Autodesk Inventor part; units mm, degrees
ref_plane "YZ Plane" through (0, 0, 0) normal (1, 0, 0) x (0, 1, 0)
ref_plane "XZ Plane" through (0, 0, 0) normal (0, 1, 0) x (-1, 0, 0)
ref_plane "XY Plane" through (0, 0, 0) normal (0, 0, 1) x (1, 0, 0)
sketch "Skizze1" plane through (0, 0, 0) normal (0, 0, 1) x (1, 0, 0)
  circle A0 centre (0, 0) radius 11
  dimension "d0" = 22
extrude "Extrusion1" add sketch "Skizze1" along normal blind 4
sketch "Skizze2" plane through (0, 0, 4) normal (0, 0, 1) x (1, 0, 0)
  circle A0 centre (0, 0) radius 11
  circle A1 centre (0, 0) radius 4
  dimension "d3" = 8
extrude "Extrusion2" add sketch "Skizze2" along normal blind 6 contours A1
sketch "Skizze3" plane through (0, 0, 10) normal (0, 0, 1) x (1, 0, 0)
  circle A0 centre (0, 0) radius 4
  circle A1 centre (0, 0) radius 2.5
  dimension "d6" = 5
extrude "Extrusion3" add sketch "Skizze3" along normal blind 20 contours A1
sketch "Skizze4" plane through (0, 0, 0) normal (0, 0, -1) x (-1, 0, 0)
  circle A0 centre (0, 0) radius 11
  line L0 (17.5, 0) -> (-17.5, 0)
  line L1 (0, -17.5) -> (0, 17.5)
  circle A1 centre (0, 0) radius 7.5
  line L2 (6.4952, -3.75) -> (0, 0)
  line L3 (0, 0) -> (-6.4952, -3.75)
  point P0 (0, 7.5)
  dimension "d9" = 15
  dimension "d10" = 120
  dimension "d11" = 120
hole "Bohrung1" at (0, 7.5, 0) at (-6.4952, -3.75, 0) at (6.4952, -3.75, 0) direction (0, 0, 1) diameter 2.459 end through all
chamfer "Fase1" distance 0.5 angle 45 1 edges at (-2.5, 0, 30)
sketch "Skizze5" plane through (0, 0, 0) normal (1, 0, 0) x (0, 1, 0)
  line L0 (-2.5, 10) -> (2.5, 10)
  line L1 (2.5, 29.5) -> (-2.5, 29.5)
  line L2 (2.5, 10) -> (2.5, 29.5)
  line L3 (0, -4.3) -> (0, 25.8)
  line L4 (2.5, 28.7) -> (2.4, 28.7)
  line L5 (2.4, 28.7) -> (2.4, 28)
  line L6 (2.4, 28) -> (2.5, 28)
  line L7 (2.5, 28) -> (2.5, 28.7)
  point P0 (0, 0)
  dimension "d31" = 18
  dimension "d32" = 0.7
  dimension "d33" = 4.8
revolve "Umdrehung1" cut sketch "Skizze5" angle 360 about axis through (0, 0, -10) along (0, 0, 1)
chamfer "Fase3" distance 1 angle 45 1 edges at (-11, 0, 4)
properties part number "13_0204_017"
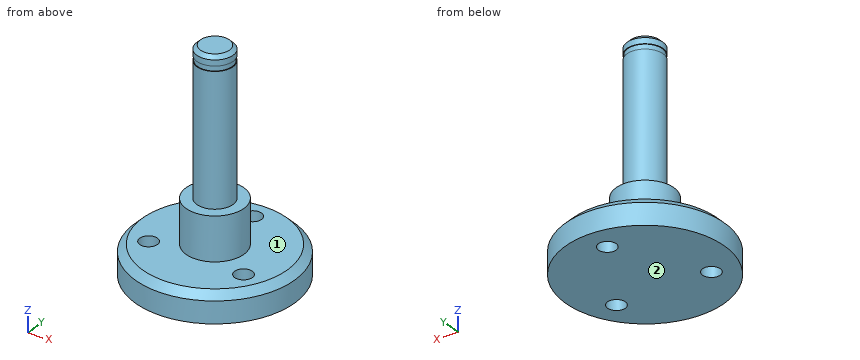
The listing builds one solid part. Answer for the finished solid, in the listing's coordinates (mm). Face numbers are marked on the shaded views. A direction names the side the tool comes from. Round coordinates to 2 decimals unless told otherwise and drop trailing zeros. Order: outer loops, then holes, each group sorted by start corner. A loop starts at its lowest first (then second) coordinate and runs counter-clockwise, first axis right, second up. Notation, with made-up numbers: (57.5, 27.5) - (116.5, 27.5) arc R28 ccw to (116.5, 66.5) - close; hole circle Ø4 at (-8.75, -22.5). An arc over 180 degrees is marked (long way). Put each result on its own line as item: value. Start each with the question number.
(1) Given P1, Ø8, axis at y = 1.5, z = 16.5, coming from the +X side; P2, Ø3, axis at x = 2.5, y = -8.5, coming from the +Z side; P3, Ø5, axis at x = 2, z = 23.5, coming from the +Y side; P4, Ø2, axis at x = -6.5, y = -3.75, coming from the -Z side, each flat-ended and moving along its own axis, determine where each tip first touches the part or whether it passes through.
(2) Find section B-B (y = 0). Give the vertices of the cut face in (x, z).
(3) Straight lines are drawn through the part: probe 1 along Y at (x, z) = (0, 1.1); probe 2 along X at (y, z) = (-3.75, 2.25); probe 3 along Z at (x, y) = (-5.25, 1.5). For each, find the intervals that lie inside material, in ascending order. Write a range as from..to.
(4) Find section D-D (z = 18.5). Give the vertices of the cut face in (x, y), plus the area to 3 significant figures.
(5) Find section C-C (z = 4.75). Give the vertices of the cut face in (x, y), plus the area to 3 significant figures.
(6) Find section A-A (x = 0). Give the vertices of the cut face in (y, z), plus the area to 3 significant figures.
(7) For the marked faces 1 and 2, determine the directions among +Z, -Z, +X, -X, +Y, -Y from which every point of the face is accessible in a straight line to the end or side of a thin tool.
Reply:
1. P1: x = 2.5
1. P2: z = 4
1. P3: y = 2.5
1. P4: through
2. outline: (-11, 0) - (11, 0) - (11, 3) - (10, 4) - (4, 4) - (4, 10) - (2.5, 10) - (2.5, 28) - (2.4, 28) - (2.4, 28.7) - (2.5, 28.7) - (2.5, 29.5) - (2, 30) - (-2, 30) - (-2.5, 29.5) - (-2.5, 28.7) - (-2.4, 28.7) - (-2.4, 28) - (-2.5, 28) - (-2.5, 10) - (-4, 10) - (-4, 4) - (-10, 4) - (-11, 3) - close
3. probe 1: -11..6.27, 8.73..11
3. probe 2: -10.34..-7.72, -5.27..5.27, 7.72..10.34
3. probe 3: 0..4
4. outline: circle Ø5 at (0, 0)
4. area: 19.6 mm^2
5. outline: circle Ø8 at (0, 0)
5. area: 50.3 mm^2
6. outline: (-11, 0) - (6.27, 0) - (6.27, 4) - (4, 4) - (4, 10) - (2.5, 10) - (2.5, 28) - (2.4, 28) - (2.4, 28.7) - (2.5, 28.7) - (2.5, 29.5) - (2, 30) - (-2, 30) - (-2.5, 29.5) - (-2.5, 28.7) - (-2.4, 28.7) - (-2.4, 28) - (-2.5, 28) - (-2.5, 10) - (-4, 10) - (-4, 4) - (-10, 4) - (-11, 3) - close; (8.73, 0) - (11, 0) - (11, 3) - (10, 4) - (8.73, 4) - close
6. area: 225 mm^2
7. face 1: +Z
7. face 2: -Z, +X, -X, +Y, -Y
